```python
from build123d import *

# Parameters (mm, degrees)
F0_R     = 12.5
F1_DEPTH = 137
F0_R_2   = 14
F2_DEPTH = 100
F0_R_3   = 16
F3_DEPTH = 25


with BuildPart() as f1:
    # F0 (on Front) → F1 (new body, symmetric)
    with BuildSketch(Plane.XZ):
        Circle(F0_R)
    extrude(amount=F1_DEPTH, both=True)

    # F0 (on Front) → F2 (join, symmetric)
    with BuildSketch(Plane.XZ):
        Circle(F0_R_2)
        Circle(F0_R, mode=Mode.SUBTRACT)
    extrude(amount=F2_DEPTH, both=True)

    # F0 (on Front) → F3 (join, symmetric)
    with BuildSketch(Plane.XZ):
        Circle(F0_R_3)
        Circle(F0_R_2, mode=Mode.SUBTRACT)
    extrude(amount=F3_DEPTH, both=True)


solid = f1.part
```
For this review, take the finished solid that the model builds, in its own axes (mm). A direction names the side the tool comes from. Give positions to 0.01 mm unless a question says otherwise; leave off trailing zeros. Loops run counter-clockwise (first coordinate to the right, second up) from the corner with the lowest first, then second, coordinate; pieces in that order, holes last. Notation, with made-up numbers: M -16.75,49.25 L 15.25,49.25 A36 cw 15.25,86.25 Z; hole C -20.75,30 d9. An arc over 180 degrees is marked long. One line per item, written item: value. Start each with the question number.
Q1. Add section B-B (z = 0). Give the boundary of the cut face in (x, y), and give its area (3 significant figures).
Q2. Add section A-A (x = 0). Give the boundary of the cut face in (y, z), and give its area (3 significant figures).
Q3. Machinability: for faces 1 (the face through (-5.3, -100, 11.5)), 2 (the face through (0, 137, 0)), 3 (the face through (12.932, 61.975, -5.362)), which of the approach directions +Z, -Z, +X, -X, +Y, -Y give a long, thin tool a straight path to every point of the face, cutting with its end or side? Answer none if there is none.
Q4. For L1, parallel to X at y = -8, z = -0.5; L2, parallel to Y at x = 14, z = 7; L3, parallel to Y at x = 0, z = 13.5, list the stretches that pass through material, from the lowest coordinate up.
Q5. Add section D-D (y = -70.5). Give the boundary of the cut face in (x, z), and give its area (3 significant figures).
Q6. Add section C-C (y = -17.5). Give the boundary of the cut face in (x, z).
Q7. Clearance check with flat-ended pins moving along their axes: pin 1 Ø1.5 at (x, y) = (3, 54.5) entering from +Z; pin 2 Ø3 at (y, z) = (-49, -11) entering from +X; pin 3 Ø4 at (x, y) = (8, -19) entering from -Z. State where each tip first meets the part, or that it passes through.
Reply:
1. outline: M -16,-25 L -14,-25 L -14,-100 L -12.5,-100 L -12.5,-137 L 12.5,-137 L 12.5,-100 L 14,-100 L 14,-25 L 16,-25 L 16,25 L 14,25 L 14,100 L 12.5,100 L 12.5,137 L -12.5,137 L -12.5,100 L -14,100 L -14,25 L -16,25 Z
1. area: 7,650 mm²
2. outline: M -137,-12.5 L -100,-12.5 L -100,-14 L -25,-14 L -25,-16 L 25,-16 L 25,-14 L 100,-14 L 100,-12.5 L 137,-12.5 L 137,12.5 L 100,12.5 L 100,14 L 25,14 L 25,16 L -25,16 L -25,14 L -100,14 L -100,12.5 L -137,12.5 Z
2. area: 7,650 mm²
3. face 1: -Y
3. face 2: +Z, -Z, +X, -X, +Y
3. face 3: +Y
4. L1: -15.99 to 15.99
4. L2: -25 to 25
4. L3: -100 to 100
5. outline: C 0,0 d28
5. area: 616 mm²
6. outline: C 0,0 d32
7. pin 1: z = 13.82
7. pin 2: x = 10.28
7. pin 3: z = -14.83
